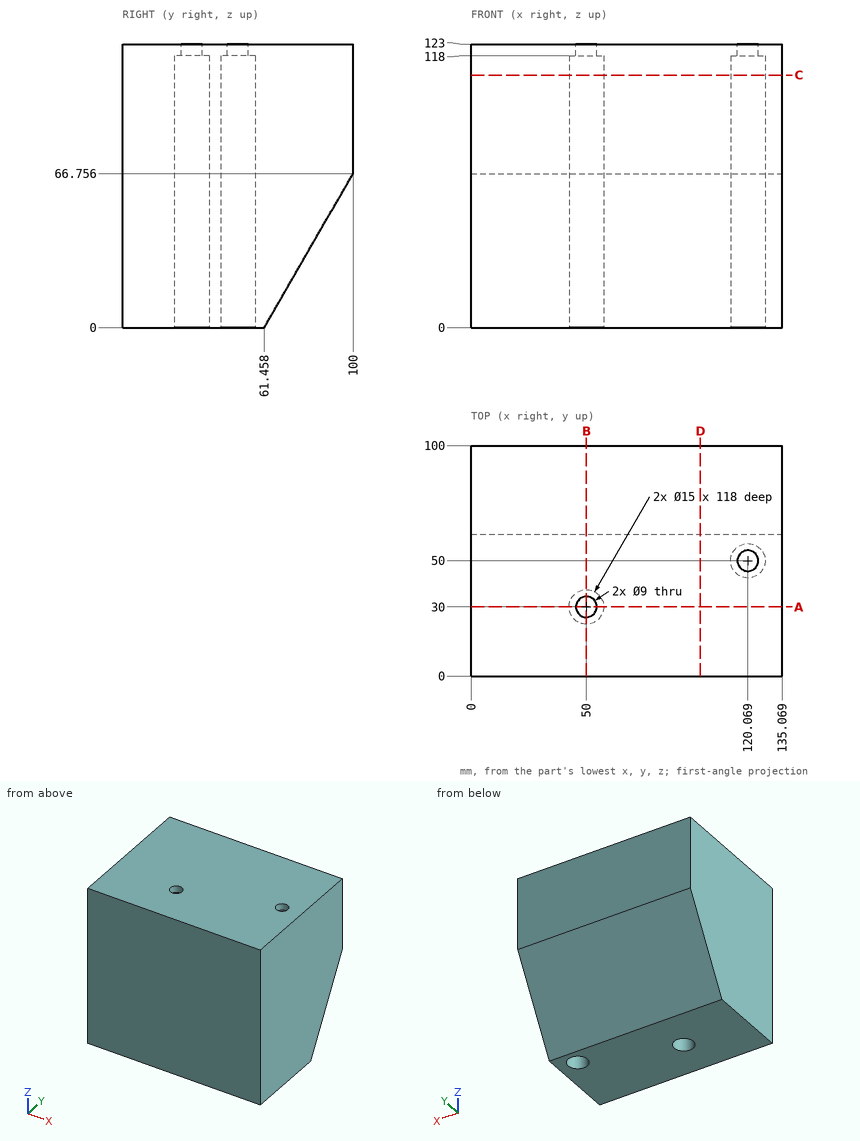
Job drawing, mm, ordinate dimensions from the low corner. One solid piece. Round coordinates to 2 decimals unless told otherwise and drop trailing zeros. Order: outer loops, then holes, each group sorted by start corner. A loop starts at its lowest first (then second) coordinate and runs counter-clockwise, first axis right, second up. Notation, with made-up numbers: (62.5, 5.5) -> (111.5, 5.5) arc R21 ccw to (111.5, 25.5) -> close; hole circle Ø2 at (52.5, 27.25). An arc over 180 degrees is marked (long way). Write item = value, one per line.
(1) Drill centre lines: L1, parallel to X at y = 24, z = 96.5; L2, parallel to Y at x = 50, z = 69.5; L3, parallel to Y at x = 53.5, z = 22 (1 decimal). Where is each one in solid material? Low to high.
Answers follow:
L1 = 0 to 45.5, 54.5 to 135.07
L2 = 0 to 22.5, 37.5 to 100
L3 = 0 to 23.4, 36.6 to 74.2
(2) Cut at A-A (y = 30). Write the cut outline in (x, z), plus the area to 3 significant figures.
Answers follow:
outline = (0, 0) -> (42.5, 0) -> (42.5, 118) -> (45.5, 118) -> (45.5, 123) -> (0, 123) -> close; (54.5, 118) -> (57.5, 118) -> (57.5, 0) -> (135.07, 0) -> (135.07, 123) -> (54.5, 123) -> close
area = 14,800 mm²
(3) Flat gauge pins, fed straight in: P1, Ø4, axis at y = 53.5, z = 99, coming from the -X side; P2, Ø13.5, axis at x = 50, y = 30, coming from the -Z side. Where does each tip first touch, or does it go through?
Answers follow:
P1 = 0
P2 = 118
(4) Cut at C-C (z = 109.5). Write the cut outline in (x, y).
Answers follow:
outline = (0, 0) -> (135.07, 0) -> (135.07, 100) -> (0, 100) -> close; hole circle Ø15 at (50, 30); hole circle Ø15 at (120.07, 50)
(5) Cut at D-D (x = 99.5). Write the cut outline in (y, z), plus the area to 3 significant figures.
Answers follow:
outline = (0, 0) -> (61.46, 0) -> (100, 66.76) -> (100, 123) -> (0, 123) -> close
area = 11,000 mm²
(6) Cut at B-B (x = 50). Write the cut outline in (y, z), plus the area to 3 significant figures.
Answers follow:
outline = (0, 0) -> (22.5, 0) -> (22.5, 118) -> (25.5, 118) -> (25.5, 123) -> (0, 123) -> close; (34.5, 118) -> (37.5, 118) -> (37.5, 0) -> (61.46, 0) -> (100, 66.76) -> (100, 123) -> (34.5, 123) -> close
area = 9,200 mm²
